The model under review builds one solid part; all positions refer to its coordinate system, in mm. A direction names the side the tool comes from. Give positions to 0.01 mm unless a question says otherwise; leave off trailing zeros. Loops run counter-clockwise (first coordinate to the right, second up) from the corner with the lowest first, then second, coordinate; pieces in that order, holes last. Notation, with made-up numbers: (-25.75, 20.25) - (15.25, 20.25) arc R16 cw to (15.25, 25.25) - close; hole circle Ø6 at (26.25, 64.25). An arc over 180 degrees is marked (long way). Return JSON: item names as keys, results as strings. Group by question number.
```python
from build123d import *

# Parameters (mm, degrees)
SKETCH2_R               = 10.75
CUT_EXTRUDE1_DEPTH      = 15
BOSS_EXTRUDE1_REACH     = 45
SKETCH3_R               = 14.75
SKETCH3_R_2             = 10.75
SKETCH4_R               = 14.75
SKETCH4_R_2             = 10.75
BOSS_EXTRUDE2_DEPTH     = 15
SKETCH5_R               = 2
CUT_EXTRUDE2_DEPTH      = 22.5
CUT_EXTRUDE2_DEPTH_BACK = 22.5
SKETCH7_R               = 2
CUT_EXTRUDE3_DEPTH      = 22.5
CUT_EXTRUDE3_DEPTH_BACK = 22.5


with BuildPart() as part:
    # Sketch1 → Revolve1 (revolve)
    with BuildSketch(Plane.XY):
        with BuildLine():
            Line((0, 21.5), (0, -21.5))
            ThreePointArc((0, -21.5), (21.5, 0), (0, 21.5))
        make_face()
    revolve(axis=Axis((0, 21.5, 0), (0, -1, 0)))

    # Sketch2 → Cut-Extrude1 (cut)
    with BuildSketch(Plane.XY.offset(21.5)):
        Circle(SKETCH2_R)
    extrude(amount=-CUT_EXTRUDE1_DEPTH, mode=Mode.SUBTRACT)

    # Sketch3 → Boss-Extrude1 (add, up to next)
    with BuildSketch(Plane.XY.offset(21.5), mode=Mode.PRIVATE) as boss_extrude1_sk1:
        Circle(SKETCH3_R)
        Circle(SKETCH3_R_2, mode=Mode.SUBTRACT)
    boss_extrude1_tool1 = extrude(boss_extrude1_sk1.sketch, amount=-BOSS_EXTRUDE1_REACH, mode=Mode.PRIVATE) - part.part
    add(boss_extrude1_tool1.solids().sort_by_distance((-14.332807, 0, 21.5))[0])

    # Sketch4 → Boss-Extrude2 (add)
    with BuildSketch(Plane.XY.offset(21.5)):
        Circle(SKETCH4_R)
        Circle(SKETCH4_R_2, mode=Mode.SUBTRACT)
    extrude(amount=BOSS_EXTRUDE2_DEPTH)

    # Sketch5 → Cut-Extrude2 (cut, two sides)
    with BuildSketch(Plane(origin=(0, 0, 0), x_dir=(1, 0, 0), z_dir=(0, 1, 0))) as cut_extrude2_sk:
        with Locations((0, -29.5)):
            Circle(SKETCH5_R)
    extrude(amount=CUT_EXTRUDE2_DEPTH, mode=Mode.SUBTRACT)
    extrude(cut_extrude2_sk.sketch, amount=-CUT_EXTRUDE2_DEPTH_BACK, mode=Mode.SUBTRACT)

    # Sketch7 → Cut-Extrude3 (cut, two sides)
    with BuildSketch(Plane(origin=(0, 0, 0), x_dir=(0, 0, -1), z_dir=(1, 0, 0))) as cut_extrude3_sk:
        with Locations((-29.5, 0)):
            Circle(SKETCH7_R)
    extrude(amount=CUT_EXTRUDE3_DEPTH, mode=Mode.SUBTRACT)
    extrude(cut_extrude3_sk.sketch, amount=-CUT_EXTRUDE3_DEPTH_BACK, mode=Mode.SUBTRACT)


solid = part.part
```
1) We need section A-A, the plane x = 0. Write out the cut boundary in (y, z).
2) For pin 1 Ø2 at (x, z) = (9.5, 4.5) entering from +Y; pin 2 Ø10 at (x, y) = (-9, -16.5) entering from -Z; pin 3 Ø10 at (y, z) = (4, -2.5) entering from +X, all flat-tipped, find the tip position at first contact; note any pin that passes through.
3) Tool access review of faces 4 (the face through (-12.627, 0.601, 27.592)), 5 (the face through (14.07, 4.43, 25.93)): name each direction out of +Z, -Z, +X, -X, +Y, -Y from which nothing blocks a thin tool from reaching the whole face with its end or side.
4) Draft analysis for pull direction Z (two halves, no side actions). For faces 1 (the face through (12.627, 0.601, 27.592)), 2 (the face through (1, -11, 36.5)), 3 (the face through (-0.434, 12.626, 31.452)), state which applies: +Z half, -Z half, draft (parallel to the pull), parting line (faces both ways), or undercut.
5) To check wall thickness, follow line 1 (X direction, y = 0, z = 24.5); line 2 (X direction, y = 11.75, z = 29.5). State the ranges of each line that lie inside material, in increasing order.
6) We need section C-C, the plane z = 29.5. Write out the cut boundary in (x, y).
7) We need section D-D, the plane y = -9.5. Write out the cut boundary in (x, z), plus the area to 3 significant figures.
Findings:
{
 "1": {"outline": "(-14.75, 15.64) arc R21.5 ccw (long way) to (14.75, 15.64) - (14.75, 27.5) - (10.75, 27.5) - (10.75, 6.5) - (-10.75, 6.5) - (-10.75, 27.5) - (-14.75, 27.5) - close; (-14.75, 31.5) - (-10.75, 31.5) - (-10.75, 36.5) - (-14.75, 36.5) - close; (10.75, 31.5) - (14.75, 31.5) - (14.75, 36.5) - (10.75, 36.5) - close"},
 "2": {"pin 1": "stops at y = 19.28", "pin 2": "stops at z = -16.49", "pin 3": "stops at x = 21.5"},
 "3": {"face 4": "+X, -X", "face 5": "+Z"},
 "4": {"face 1": "undercut", "face 2": "+Z half", "face 3": "undercut"},
 "5": {"line 1": "x = -14.75 to -10.75, 10.75 to 14.75", "line 2": "x = -8.92 to -2, 2 to 8.92"},
 "6": {"outline": "(-14.61, -2) arc R14.75 ccw to (-2, -14.61) - (-2, -10.56) arc R10.75 cw to (-10.56, -2) - close; (-14.61, 2) - (-10.56, 2) arc R10.75 cw to (-2, 10.56) - (-2, 14.61) arc R14.75 ccw to start; (2, -14.61) arc R14.75 ccw to (14.61, -2) - (10.56, -2) arc R10.75 cw to (2, -10.56) - close; (2, 10.56) arc R10.75 cw to (10.56, 2) - (14.61, 2) arc R14.75 ccw to (2, 14.61) - close"},
 "7": {"outline": "(-11.28, 15.64) arc R19.29 ccw (long way) to (11.28, 15.64) - (11.28, 36.5) - (5.03, 36.5) - (5.03, 6.5) - (-5.03, 6.5) - (-5.03, 36.5) - (-11.28, 36.5) - close", "area": "1,280 mm^2"}
}
